from build123d import *

# Parameters (mm, degrees)
SKETCH1_W           = 25.4
SKETCH1_H           = 25.4
SKETCH1_W_2         = 19.05
SKETCH1_H_2         = 19.05
BOSS_EXTRUDE1_DEPTH = 101.6
CUT_EXTRUDE1_REACH  = 107.494


with BuildPart() as part:
    # Sketch1 → Boss-Extrude1 (new body)
    with BuildSketch(Plane.XY):
        Rectangle(SKETCH1_W, SKETCH1_H)
        Rectangle(SKETCH1_W_2, SKETCH1_H_2, mode=Mode.SUBTRACT)
    extrude(amount=BOSS_EXTRUDE1_DEPTH)

    # Cut-Extrude1: up to this face of the body (flat: up to its plane)
    cut_extrude1_end = Plane(part.part.faces().sort_by_distance((-12.7, 0, 50.8))[0])
    # Sketch2 → Cut-Extrude1 (cut, up to the picked face)
    with BuildSketch(Plane(origin=(12.7, 0, 0), x_dir=(0, 0, -1), z_dir=(1, 0, 0)), mode=Mode.PRIVATE) as cut_extrude1_sk1:
        Polygon((-101.6, 12.7), (-101.6, -12.7), (-76.2, 12.7), align=None)
    cut_extrude1_tool1 = split(extrude(cut_extrude1_sk1.sketch, amount=-CUT_EXTRUDE1_REACH, mode=Mode.PRIVATE), bisect_by=cut_extrude1_end, keep=Keep.BOTH, mode=Mode.PRIVATE)
    # Sketch2 → Cut-Extrude1 (cut, up to the picked face)
    with BuildSketch(Plane(origin=(12.7, 0, 0), x_dir=(0, 0, -1), z_dir=(1, 0, 0)), mode=Mode.PRIVATE) as cut_extrude1_sk2:
        Polygon((-25.4, 12.7), (0, -12.7), (0, 12.7), align=None)
    cut_extrude1_tool2 = split(extrude(cut_extrude1_sk2.sketch, amount=-CUT_EXTRUDE1_REACH, mode=Mode.PRIVATE), bisect_by=cut_extrude1_end, keep=Keep.BOTH, mode=Mode.PRIVATE)
    add(cut_extrude1_tool1.solids().sort_by(Axis((12.7, 4.233333, 93.133333), (-1, 0, 0)))[0], mode=Mode.SUBTRACT)
    add(cut_extrude1_tool2.solids().sort_by(Axis((12.7, 4.233333, 8.466667), (-1, 0, 0)))[0], mode=Mode.SUBTRACT)


solid = part.part
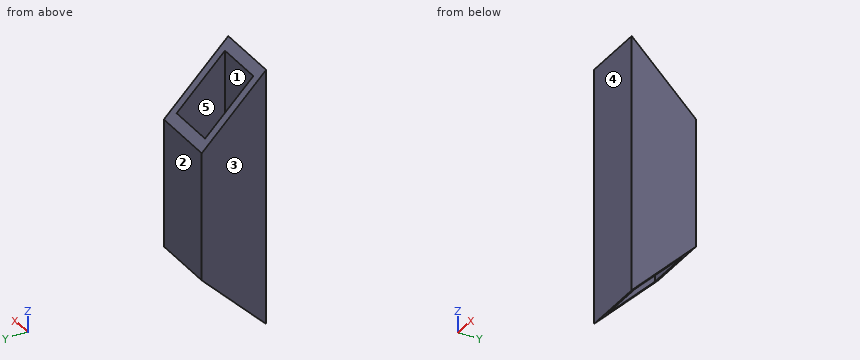
Design review of the part built by this model. Coordinates are the model's own, in mm. Face numbers are marked on the shaded views. A direction names the side the tool comes from. Round coordinates to 2 decimals unless told otherwise and drop trailing zeros. Loops run counter-clockwise (first coordinate to the right, second up) from the corner with the lowest first, then second, coordinate; pieces in that order, holes last. Notation, with made-up numbers: (82, -10.5) -> (108, -10.5) arc R21 ccw to (108, 21.5) -> close; hole circle Ø9 at (37, 64.25). An arc over 180 degrees is marked (long way). Use one line per item in the form item = value. Start each with the question number.
Q1. Machinability: for the marked faces 1 and 2, which of the approach directions +Z, -Z, +X, -X, +Y, -Y give a long, thin tool a straight path to every point of the face, cutting with its end or side? Answer none if there is none.
Q2. Wall thickness on line 1 along X through (y, z) = (-1.25, 45) (3 decimals); line 2 along Y through (x, z) = (-8.75, 90) (3 decimals): over which ranges is each line inside the solid? List them lowest first. Write a range as [from, to].
Q3. We need section C-C on x = 7.5. Give the boundary of the cut face in (y, z) (3 decimals).
Q4. We need section A-A on y = 6.5. Give the boundary of the cut face in (x, z) (3 decimals), then the cut area to 3 significant figures.
Q5. Draft analysis for pull direction X (two halves, no side actions). For the marked faces 3, 4 and 5, state which applies: +X half, -X half, draft (parallel to the pull), parting line (faces both ways), or undercut.
Q6. We need section D-D on z = 81. Give the boundary of the cut face in (x, y) (3 decimals).
Q7. We need section B-B on z = 49. Give the boundary of the cut face in (x, y) (3 decimals), then the cut area to 3 significant figures.
Q8. For pin 1 Ø3 at (x, y) = (9.5, -1.5) entering from -Z, flat-tipped, find the tip position at first contact; note if it passes through.
Calculated:
q1.face_1 = +Z, -Z
q1.face_2 = +Z, -Z, +X, -X, +Y
q2.line_1 = [-12.7, -9.525], [9.525, 12.7]
q2.line_2 = [-12.7, -9.525]
q3.outline = (-12.7, 0) -> (-9.525, 3.175) -> (-9.525, 98.425) -> (-12.7, 101.6) -> close; (9.525, 22.225) -> (12.7, 25.4) -> (12.7, 76.2) -> (9.525, 79.375) -> close
q4.outline = (-12.7, 19.2) -> (-9.525, 19.2) -> (-9.525, 82.4) -> (-12.7, 82.4) -> close; (9.525, 19.2) -> (12.7, 19.2) -> (12.7, 82.4) -> (9.525, 82.4) -> close
q4.area = 401 mm²
q5.face_3 = -X half
q5.face_4 = draft
q5.face_5 = undercut
q6.outline = (-12.7, -12.7) -> (12.7, -12.7) -> (12.7, 7.9) -> (9.525, 7.9) -> (9.525, -9.525) -> (-9.525, -9.525) -> (-9.525, 7.9) -> (-12.7, 7.9) -> close
q7.outline = (-12.7, -12.7) -> (12.7, -12.7) -> (12.7, 12.7) -> (-12.7, 12.7) -> close; hole (-9.525, -9.525) -> (9.525, -9.525) -> (9.525, 9.525) -> (-9.525, 9.525) -> close
q7.area = 282 mm²
q8.pin_1 = 9.7
